CAD build for the part. Positions are in the model's coordinates, mm. Give positions to 0.01 mm unless a question says otherwise; leave off trailing zeros. Order: outer loops, then holes, each group sorted by start corner. A loop starts at its lowest first (then second) coordinate and runs counter-clockwise, first axis right, second up. Notation, with made-up numbers: (-11.75, 60.5) -> (29.25, 60.5) arc R27 cw to (29.25, 99.5) -> close; hole circle Ø10 at (-29, -5). An arc over 180 degrees is marked (long way). Use one line per item in the form item = value. Start each with the question number.
1) Cut at A-A, the plane y = 4.85. Give the cut face in (x, z).
2) Cut at B-B, the plane z = -2.5. Give the cut face in (x, y).
3) Probe line 1 (X direction, y = 4.9, z = -3); line 2 (Z direction, x = -2.5, y = 4.75). List the from-to ranges inside material, lowest first.
4) Cut at C-C, the plane x = -0.75. Give the cut face in (y, z), and give its area (3 significant figures).
from build123d import *

# Parameters (mm, degrees)
SKETCH027_W  = 7.5
SKETCH027_H  = 0.5
PAD011_DEPTH = 5
SKETCH028_W  = 1
SKETCH028_H  = 0.5
PAD012_DEPTH = 3.5
FILLET006_R  = 0.45


with BuildPart() as part:
    # Sketch027 → Pad011 (new body)
    with BuildSketch(Plane.XY):
        with Locations((0, 4.92)):
            Rectangle(SKETCH027_W, SKETCH027_H)
    extrude(amount=PAD011_DEPTH)

    # Sketch028 (on Face5 of Pad011) → Pad012 (join)
    with BuildSketch(Plane(origin=(0, 0, 0), x_dir=(1, 0, 0), z_dir=(0, 0, -1))):
        with Locations((0, -4.92)):
            Rectangle(SKETCH028_W, SKETCH028_H)
    extrude(amount=PAD012_DEPTH)

    # Fillet006
    fillet006_edges = [part.edges().sort_by_distance(p)[0] for p in [
        (0.5, 4.92, -3.5),
        (-0.5, 4.92, -3.5),
    ]]
    fillet(fillet006_edges, radius=FILLET006_R)


solid = part.part
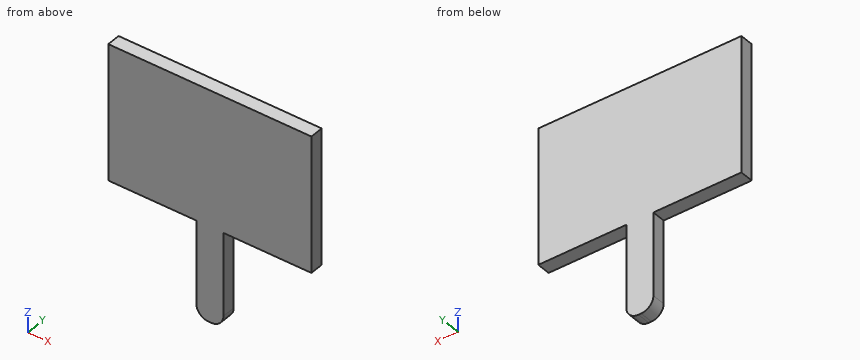
Result:
q1.outline = (-3.75, 0) -> (-0.5, 0) -> (-0.5, -3.05) arc R0.45 ccw to (-0.05, -3.5) -> (0.05, -3.5) arc R0.45 ccw to (0.5, -3.05) -> (0.5, 0) -> (3.75, 0) -> (3.75, 5) -> (-3.75, 5) -> close
q2.outline = (-0.5, 4.67) -> (0.5, 4.67) -> (0.5, 5.17) -> (-0.5, 5.17) -> close
q3.line_1 = -0.5 to 0.5
q3.line_2 = 0 to 5
q4.outline = (4.67, 0) -> (5.17, 0) -> (5.17, 5) -> (4.67, 5) -> close
q4.area = 2.50 mm²
